Could you check a few things on this model? Use its own coordinates, in mm. Face numbers are marked on the shaded views. A direction names the side the tool comes from. Give positions to 0.01 mm unless a question says otherwise; leave off trailing zeros. Write each loop counter-clockwise with the first axis right and the second up, starting at its lowest first coordinate (ties: lowest second). Pieces come first, ordered by that corner, then holes. Notation, with made-up numbers: (62, 31) - (108, 31) arc R19 cw to (108, 61) - close; hole circle Ø1 at (26.5, 28.25). An arc over 180 degrees is marked (long way). Use one line per item in the form item = value.
```python
from build123d import *

# Parameters (mm, degrees)
F1_DEPTH = 63.5
F0_W     = 25.4
F0_H     = 19.05
F2_DEPTH = 25.4
F4_R     = 6.35


with BuildPart() as f1:
    # F0 (on Front) → F1 (new body, symmetric)
    with BuildSketch(Plane.XZ):
        Polygon((-41.275, -9.525), (41.275, -9.525), (41.275, 9.525), (22.225, 9.525), (-41.275, 9.525), align=None)
    extrude(amount=F1_DEPTH, both=True)

    # F0 (on Front) → F2 (join, symmetric)
    with BuildSketch(Plane.XZ):
        with BuildLine():
            Line((22.225, 9.525), (41.275, 9.525))
            Line((41.275, 9.525), (41.275, 27.0002))
            ThreePointArc((41.275, 27.0002), (45.9246798487, 38.2255201513), (57.15, 42.8752))
            Line((57.15, 42.8752), (60.325, 42.8752))
            Line((60.325, 42.8752), (60.325, 61.9252))
            Line((60.325, 61.9252), (57.15, 61.9252))
            add(Edge.make_bspline(
                [(56.3590284094, 61.916242), (56.6228100042, 61.9198399191), (56.8864704365, 61.9228263572), (57.15, 61.9252)],
                knots=[110.8800501916, 110.8800501916, 110.8800501916, 110.8800501916, 111.5045361635, 111.5045361635, 111.5045361635, 111.5045361635], degree=3))
            ThreePointArc((56.3590284094, 61.916242), (32.176210662, 51.414652095), (22.225, 27.0002))
            Line((22.225, 27.0002), (22.225, 9.525))
        make_face()
        with Locations((73.025, 52.4002)):
            Rectangle(F0_W, F0_H)
    extrude(amount=F2_DEPTH, both=True)

    # F0 (on Front) → F3 (revolve)
    with BuildSketch(Plane.XZ):
        Polygon((85.725, 61.9252), (85.725, 42.8752), (85.725, 38.1), (111.125, 38.1), (111.125, 66.675), (85.725, 66.675), align=None)
    revolve(axis=Axis((85.725, 0, 52.3875), (0, 0, 1)))

    # F4
    f4_edges = [f1.edges().sort_by_distance(p)[0] for p in [
        (41.275, -63.5, 0),
        (-41.275, -63.5, 0),
        (-41.275, 63.5, 0),
        (41.275, 63.5, 0),
    ]]
    fillet(f4_edges, radius=F4_R)


solid = f1.part
```
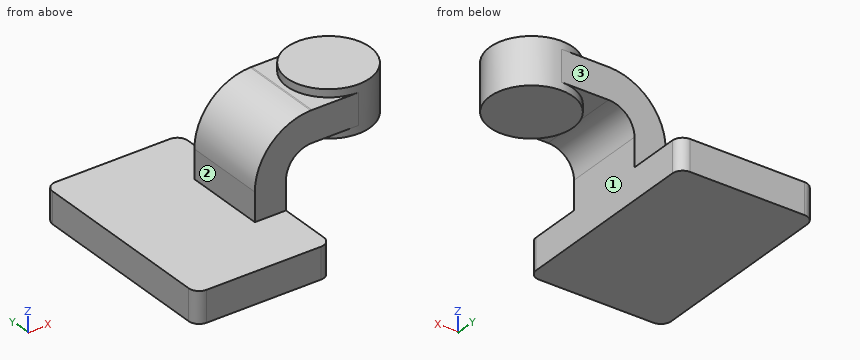
1. Imagine slicing it at C-C, the plane x = 7.5. List the corners of the cut face in (y, z) for me (3 decimals), and give its area (3 significant figures).
Response values:
outline = (-63.5, -9.525) - (63.5, -9.525) - (63.5, 9.525) - (-63.5, 9.525) - close
area = 2,420 mm²
2. Which directions (+Z, -Z, +X, -X, +Y, -Y) give clear straight access to the entire face, cutting with the end or side of a thin tool? Please do the marked faces 1, 2 and 3.
Response values:
face_1 = -Z, +X, +Y, -Y
face_2 = +Z, -X, +Y, -Y
face_3 = +Z, +X, -X, +Y
3. Imagine slicing it at B-B, the plane y = -46. List the corners of the cut face in (x, z) for me (3 decimals).
Response values:
outline = (-41.275, -9.525) - (41.275, -9.525) - (41.275, 9.525) - (-41.275, 9.525) - close
4. If I drill on line 1 (Y direction, x = 27, z = 25.5); line 2 (Z direction, x = 33, y = 39.5) (3 decimals); line 3 (X direction, y = -35, z = -3) (3 decimals), over which ranges is the centre line in solid material (lowest first)? Write a range as from..to.
Response values:
line_1 = -25.4..25.4
line_2 = -9.525..9.525
line_3 = -41.275..41.275
5. Imagine slicing it at A-A, the plane z = 6.5. List the corners of the cut face in (x, y) for me (3 decimals).
Response values:
outline = (-41.275, -57.15) arc R6.35 ccw to (-34.925, -63.5) - (34.925, -63.5) arc R6.35 ccw to (41.275, -57.15) - (41.275, 57.15) arc R6.35 ccw to (34.925, 63.5) - (-34.925, 63.5) arc R6.35 ccw to (-41.275, 57.15) - close
6. For pin 1 (8 mm diameter, centred on x = -22.5, y = -44, fed in from +Z) (3 decimals); pin 2 (8.5 mm diameter, centred on y = 4, z = 22, fed in from -X) (3 decimals); pin 3 (11 mm diameter, centred on y = 27.5, z = 12, fed in from +X) (3 decimals), each with a flat end and sliding along its axis, tell me the tip position at first contact or that it passes through.
Response values:
pin_1 = 9.525
pin_2 = 22.225
pin_3 = 41.275
